Model file for the job. Use its own axes, mm. Face numbers are marked on the shaded views. A direction names the side the tool comes from. Round coordinates to 2 decimals unless told otherwise and drop trailing zeros. Write each loop counter-clockwise with the first axis right and the second up, starting at its lowest first coordinate (ties: lowest second). Pieces come first, ordered by that corner, then holes. Notation, with made-up numbers: (78, 32.5) - (126, 32.5) arc R29 ccw to (126, 59.5) - close; hole circle Ø6 at (63.5, 69). An arc over 180 degrees is marked (long way). One line per item, written item: value.
from build123d import *

# Parameters (mm, degrees)
BOX088_W                = 80
BOX088_H                = 20
BOX088_DEPTH            = 11
BOX089_W                = 34
BOX089_H                = 20
BOX089_DEPTH            = 10
BOX087_W                = 11
BOX087_H                = 20
BOX087_DEPTH            = 76
FILLET001006007031013_R = 5
FILLET001006007031014_R = 3
CHAMFER_SIZE2           = 22
CHAMFER_SIZE            = 19.99
CHAMFER011006013_SIZE2  = 19.99
CHAMFER011006013_SIZE   = 40


with BuildPart() as cube:
    # Box088 → Box088 (new body)
    with BuildSketch(Plane.XY):
        with Locations((40, 10)):
            Rectangle(BOX088_W, BOX088_H)
    extrude(amount=BOX088_DEPTH)


with BuildPart() as box089:
    # Box089 → Box089 (new body)
    with BuildSketch(Plane(origin=(-23, 0, 64.5), x_dir=(1, 0, 0), z_dir=(0, 0, 1))):
        with Locations((17, 10)):
            Rectangle(BOX089_W, BOX089_H)
    extrude(amount=BOX089_DEPTH)


with BuildPart() as chamfer011006013:
    # Box087 → Box087 (new body)
    with BuildSketch(Plane.XY):
        with Locations((5.5, 10)):
            Rectangle(BOX087_W, BOX087_H)
    extrude(amount=BOX087_DEPTH)

    # Fusion: union Cube, Box089
    add(cube.part)
    add(box089.part)

    # Fillet001006007031013
    fillet001006007031013_edges = [chamfer011006013.edges().sort_by_distance(p)[0] for p in [
        (11, 10, 11),
        (0, 10, 0),
    ]]
    fillet(fillet001006007031013_edges, radius=FILLET001006007031013_R)

    # Fillet001006007031014
    fillet001006007031014_edges = [chamfer011006013.edges().sort_by_distance(p)[0] for p in [
        (11, 10, 76),
    ]]
    fillet(fillet001006007031014_edges, radius=FILLET001006007031014_R)

    # Chamfer
    chamfer_edges = [chamfer011006013.edges().sort_by_distance(p)[0] for p in [
        (-23, 0, 69.5),
    ]]
    chamfer_side = chamfer011006013.faces().sort_by_distance((-23, 10, 69.5))[0]
    chamfer(chamfer_edges, length=CHAMFER_SIZE, length2=CHAMFER_SIZE2, reference=chamfer_side)

    # Chamfer011006013
    chamfer011006013_edges = [chamfer011006013.edges().sort_by_distance(p)[0] for p in [
        (80, 0, 5.5),
    ]]
    chamfer011006013_side = chamfer011006013.faces().sort_by_distance((-0.5, 0, 73.38928))[0]
    chamfer(chamfer011006013_edges, length=CHAMFER011006013_SIZE, length2=CHAMFER011006013_SIZE2, reference=chamfer011006013_side)


solid = chamfer011006013.part
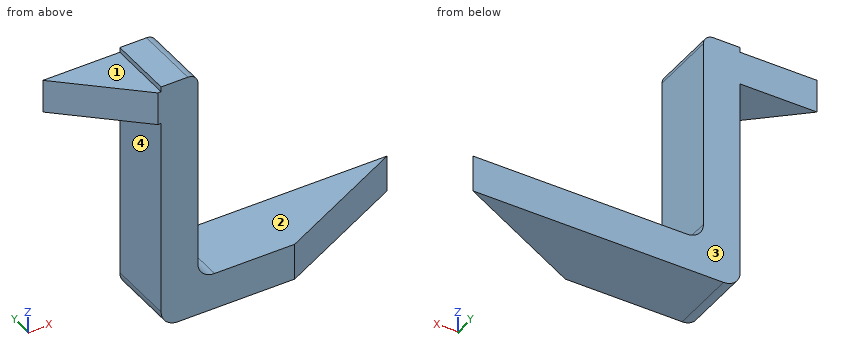
1. Band-saw the part on D-D on y = 17.5. Write the cut outline in (x, z).
Report:
outline: (-20.26, 64.5) - (0, 64.5) - (0, 5) arc R5 ccw to (5, 0) - (75.02, 0) - (75.02, 11) - (16, 11) arc R5 cw to (11, 16) - (11, 73) arc R3 ccw to (8, 76) - (0, 76) - (0, 74.5) - (-20.26, 74.5) - close
2. Drop flat-ended pins along their axis: pin 1 (10 mm diameter, centred on x = 36.5, y = 5.5, fed in from +Z); pin 2 (12 mm diameter, centred on x = 67, y = 7, fed in from -Z); pin 3 (10 mm diameter, centred on x = -16.5, y = 14, fed in from -Z); pin 4 (2 mm diameter, centred on x = -5, y = 6.5, fed in from +Z). Give the stop position or say it passes through.
Report:
pin 1: z = 11
pin 2: z = 0
pin 3: z = 64.5
pin 4: z = 74.5
3. Band-saw the part on B-B on x = 24. Write the cut outline in (y, z).
Report:
outline: (0, 0) - (20, 0) - (20, 11) - (0, 11) - close
4. Wall check: probe 1 along X at (y, z) = (2.25, 50.5); probe 2 along Z at (x, y) = (4.5, 8.5). Give the ranges that are in metal, low to high. Write a range as [from, to].
Report:
probe 1: [0, 11]
probe 2: [0.03, 76]
5. Band-saw the part on A-A on y = 5.75. Write the cut outline in (x, z), plus the area to 3 significant figures.
Report:
outline: (-7.33, 64.5) - (0, 64.5) - (0, 5) arc R5 ccw to (5, 0) - (51.51, 0) - (51.51, 11) - (16, 11) arc R5 cw to (11, 16) - (11, 73) arc R3 ccw to (8, 76) - (0, 76) - (0, 74.5) - (-7.33, 74.5) - close
area: 1,350 mm²
6. Band-saw the part on C-C on z = 50. Write the cut outline in (x, y).
Report:
outline: (0, 0) - (11, 0) - (11, 20) - (0, 20) - close
7. Tool access for the marked faces 1, 2, 3 and 4: list every direction of +Z, -Z, +X, -X, +Y, -Y with a clear straight run to the whole face (end or side of a thin tool).
Report:
face 1: +Z, -X, +Y, -Y
face 2: +Z, +X, +Y, -Y
face 3: +Z, -Z, +X, -X, +Y
face 4: -Z, -X, +Y, -Y
